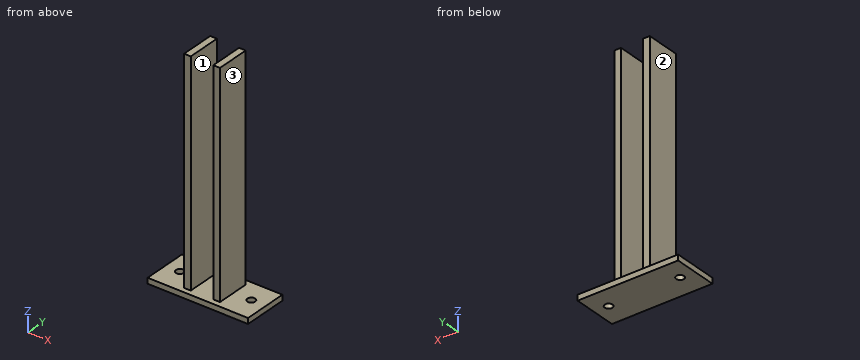
```python
from build123d import *

# Parameters (mm, degrees)
F0_W     = 40
F0_H     = 5
F1_DEPTH = 90
F2_W     = 6
F2_H     = 30.4702166427
F2_H_2   = 30
F3_DEPTH = 200
F5_D     = 7


# Not quite as in the source:
# - a feature names something its author has since deleted; it is built from what else it names


with BuildPart() as f1:
    # F0 (on Right) → F1 (new body)
    with BuildSketch(Plane.YZ):
        with Locations((-0.72813743, 2.5)):
            Rectangle(F0_W, F0_H)
    extrude(amount=F1_DEPTH)

    # F2 (on Top) → F3 (join)
    with BuildSketch(Plane.XY):
        with Locations((32, -0.7447636027)):
            Rectangle(F2_W, F2_H)
        with Locations((58, -0.72813743)):
            Rectangle(F2_W, F2_H_2)
    extrude(amount=F3_DEPTH)

    # F5 (through all)
    with Locations(Plane(origin=(0, 0, 0), x_dir=(1, 0, 0), z_dir=(0, 0, -1))):
        with Locations((13, 0), (77, 0)):
            Hole(F5_D / 2)


solid = f1.part
```
Can you work these out from the model? Positions are in its coordinate system, mm. Face numbers are marked on the shaded views. A direction names the side the tool comes from. Round coordinates to 2 decimals unless told otherwise and drop trailing zeros. Loops run counter-clockwise (first coordinate to the right, second up) from the corner with the lowest first, then second, coordinate; pieces in that order, holes last.
Item 1: Please list where these lines run through material, in increasing order: L1, parallel to X at y = 0, z = 169.5; L2, parallel to Y at x = 77, z = 1; L3, parallel to Z at x = 21, y = -7.5.
Item 2: Suppose I cut it at A-A, the plane x = 13. Write out the boundary of the cut face in (y, z).
Item 3: Suppose I cut it at B-B, the plane y = 0. Write out the boundary of the cut face in (x, z), then the cut area to 3 significant figures.
Item 4: Which directions (+Z, -Z, +X, -X, +Y, -Y) give clear straight access to the entire face, cutting with the end or side of a thin tool? Please do the marked faces 1, 2 and 3.
Item 5: Suppose I cut it at D-D, the plane x = 57. Write out the boundary of the cut face in (y, z), then the cut area to 3 significant figures.
Item 6: Will these pins go through, and if not, where does the flat tip stop? pin 1 Ø3 at (x, z) = (32, 96.5) entering from -Y; pin 2 Ø3 at (y, z) = (0, 70) entering from +X; pin 3 Ø11 at (x, y) = (77, 0) entering from +Z; pin 4 Ø4 at (x, y) = (13, 0) entering from -Z.
Item 7: Suppose I cut it at C-C, the plane z = 74. Write out the boundary of the cut face in (x, y), then the cut area to 3 significant figures.
Reported:
1. L1: x = 29 to 35, 55 to 61
1. L2: y = -20.73 to -3.5, 3.5 to 19.27
1. L3: z = 0 to 5
2. outline: (-20.73, 0) - (-3.5, 0) - (-3.5, 5) - (-20.73, 5) - close; (3.5, 0) - (19.27, 0) - (19.27, 5) - (3.5, 5) - close
3. outline: (0, 0) - (9.5, 0) - (9.5, 5) - (0, 5) - close; (16.5, 0) - (73.5, 0) - (73.5, 5) - (61, 5) - (61, 200) - (55, 200) - (55, 5) - (35, 5) - (35, 200) - (29, 200) - (29, 5) - (16.5, 5) - close; (80.5, 0) - (90, 0) - (90, 5) - (80.5, 5) - close
3. area: 2,720 mm2
4. face 1: +Z, +Y, -Y
4. face 2: +Z, -X, +Y, -Y
4. face 3: +Z, +X, +Y, -Y
5. outline: (-20.73, 0) - (19.27, 0) - (19.27, 5) - (14.27, 5) - (14.27, 200) - (-15.73, 200) - (-15.73, 5) - (-20.73, 5) - close
5. area: 6,050 mm2
6. pin 1: stops at y = -15.98
6. pin 2: stops at x = 61
6. pin 3: stops at z = 5
6. pin 4: passes through
7. outline: (29, -15.98) - (35, -15.98) - (35, 14.49) - (29, 14.49) - close; (55, -15.73) - (61, -15.73) - (61, 14.27) - (55, 14.27) - close
7. area: 363 mm2
